```python
from build123d import *

# Parameters (mm, degrees)
CROQUIS2_R                = 19
SALIENTE_EXTRUIR1_DEPTH   = 39
CROQUIS3_W                = 25
CROQUIS3_H                = 35
SALIENTE_EXTRUIR2_DEPTH   = 53
CROQUIS4_R                = 3
CORTAR_EXTRUIR1_DEPTH     = 73.953752474
REDONDEO1_R               = 5
MATRIZC2_START            = 2
MATRIZC2_DEPTH            = 9.9999999
MATRIZC2_START_2          = 18.0000001
MATRIZC2_2_DEPTH          = 6.298293978
MATRIZC2_START_3          = 11.9999999
MATRIZC2_3_DEPTH          = 25.0000001
MATRIZC2_START_4          = -12.5
MATRIZC2_4_OUTLINE_R      = 3
MATRIZC2_4_DEPTH          = 25
MATRIZC2_5_OUTLINE_R      = 3
MATRIZC2_5_DEPTH          = 25
TALADRO_ROSCADO_3_4_102_D = 16.66748


with BuildPart() as part:
    # Croquis2 → Saliente-Extruir1 (new body)
    with BuildSketch(Plane(origin=(0, 0, 0), x_dir=(1, 0, 0), z_dir=(0, 1, 0))):
        with Locations(Location((0, 0, 0), (0, 0, 270))):
            Circle(CROQUIS2_R)
    extrude(amount=SALIENTE_EXTRUIR1_DEPTH)

    # Croquis3 → Saliente-Extruir2 (add)
    with BuildSketch(Plane.XY):
        with Locations((0, 19.5)):
            Rectangle(CROQUIS3_W, CROQUIS3_H)
    extrude(amount=SALIENTE_EXTRUIR2_DEPTH)

    # Croquis4 → Cortar-Extruir1 (cut, through all)
    with BuildSketch(Plane(origin=(12.5, 0, 0), x_dir=(0, 0, -1), z_dir=(1, 0, 0))):
        with Locations((-36, 15)):
            Circle(CROQUIS4_R)
        Polygon((-53, 27.185045424), (-53, 37), (-36, 37), align=None)
    extrude(amount=-CORTAR_EXTRUIR1_DEPTH, mode=Mode.SUBTRACT)

    # Redondeo1
    redondeo1_edges = [part.edges().sort_by_distance(p)[0] for p in [
        (12.5, 14.592522712, 53),
        (-12.5, 14.592522712, 53),
        (0, 27.185045424, 53),
        (0, 37, 36),
        (12.5, 19.5, 14.309088021),
        (-12.5, 19.5, 14.309088021),
    ]]
    fillet(redondeo1_edges, radius=REDONDEO1_R)

    # MatrizC2: read off the stored shape, not the designer's step
    # MatrizC2 outline → MatrizC2 (add)
    with BuildSketch(Plane(origin=(0, 0, 0), x_dir=(1, 0, 0), z_dir=(0, 1, 0)).offset(MATRIZC2_START)):
        with BuildLine():
            Line((-42.149346401, 32.995190528), (-49.649346401, 20.004809472))
            ThreePointArc((-49.649346401, 20.004809472), (-50.148848513, 16.210714247), (-47.819219382, 13.174682453))
            Line((-47.819219382, 13.174682453), (-18.642033731, -3.670773537))
            ThreePointArc((-18.642033731, -3.670773537), (-16.454482672, 9.5), (-6.142033731, 17.979861558))
            Line((-6.142033731, 17.979861558), (-35.319219382, 34.825317547))
            ThreePointArc((-35.319219382, 34.825317547), (-39.113314608, 35.32481966), (-42.149346401, 32.995190528))
        make_face()
        with BuildLine():
            ThreePointArc((6.142033731, 17.979861558), (16.454482672, 9.5), (18.642033731, -3.670773537))
            Line((18.642033731, -3.670773537), (47.819219382, 13.174682453))
            ThreePointArc((47.819219382, 13.174682453), (50.148848513, 16.210714247), (49.649346401, 20.004809472))
            Line((49.649346401, 20.004809472), (42.149346401, 32.995190528))
            ThreePointArc((42.149346401, 32.995190528), (39.113314608, 35.32481966), (35.319219382, 34.825317547))
            Line((35.319219382, 34.825317547), (6.142033731, 17.979861558))
        make_face()
    extrude(amount=MATRIZC2_DEPTH)

    # MatrizC2 2 outline → MatrizC2 2 (add)
    with BuildSketch(Plane(origin=(0, 0, 0), x_dir=(1, 0, 0), z_dir=(0, 1, 0)).offset(MATRIZC2_START_2)):
        with BuildLine():
            Line((-42.149346401, 32.995190528), (-49.649346401, 20.004809472))
            ThreePointArc((-49.649346401, 20.004809472), (-50.148848513, 16.210714247), (-47.819219382, 13.174682453))
            Line((-47.819219382, 13.174682453), (-18.642033731, -3.670773537))
            ThreePointArc((-18.642033731, -3.670773537), (-16.454482672, 9.5), (-6.142033731, 17.979861558))
            Line((-6.142033731, 17.979861558), (-35.319219382, 34.825317547))
            ThreePointArc((-35.319219382, 34.825317547), (-39.113314608, 35.32481966), (-42.149346401, 32.995190528))
        make_face()
        with BuildLine():
            ThreePointArc((6.142033731, 17.979861558), (16.454482672, 9.5), (18.642033731, -3.670773537))
            Line((18.642033731, -3.670773537), (47.819219382, 13.174682453))
            ThreePointArc((47.819219382, 13.174682453), (50.148848513, 16.210714247), (49.649346401, 20.004809472))
            Line((49.649346401, 20.004809472), (42.149346401, 32.995190528))
            ThreePointArc((42.149346401, 32.995190528), (39.113314608, 35.32481966), (35.319219382, 34.825317547))
            Line((35.319219382, 34.825317547), (6.142033731, 17.979861558))
        make_face()
    extrude(amount=MATRIZC2_2_DEPTH)

    # MatrizC2 3 outline → MatrizC2 3 (add)
    with BuildSketch(Plane(origin=(0, 0, 0), x_dir=(1, 0, 0), z_dir=(0, 1, 0)).offset(MATRIZC2_START_3)):
        with BuildLine():
            Line((-42.149346401, 32.995190528), (-49.649346401, 20.004809472))
            ThreePointArc((-49.649346401, 20.004809472), (-50.148848513, 16.210714247), (-47.819219382, 13.174682453))
            Line((-47.819219382, 13.174682453), (-18.642033731, -3.670773537))
            ThreePointArc((-18.642033731, -3.670773537), (-16.454482672, 9.5), (-6.142033731, 17.979861558))
            Line((-6.142033731, 17.979861558), (-35.319219382, 34.825317547))
            ThreePointArc((-35.319219382, 34.825317547), (-39.113314608, 35.32481966), (-42.149346401, 32.995190528))
        make_face()
        with BuildLine():
            ThreePointArc((6.142033731, 17.979861558), (16.454482672, 9.5), (18.642033731, -3.670773537))
            Line((18.642033731, -3.670773537), (47.819219382, 13.174682453))
            ThreePointArc((47.819219382, 13.174682453), (50.148848513, 16.210714247), (49.649346401, 20.004809472))
            Line((49.649346401, 20.004809472), (42.149346401, 32.995190528))
            ThreePointArc((42.149346401, 32.995190528), (39.113314608, 35.32481966), (35.319219382, 34.825317547))
            Line((35.319219382, 34.825317547), (6.142033731, 17.979861558))
        make_face()
    extrude(amount=MATRIZC2_3_DEPTH)

    # MatrizC2 4 outline → MatrizC2 4 (cut)
    with BuildSketch(Plane(origin=(0, 0, 0), x_dir=(0.8660254037844362, 0, -0.5000000000000042), z_dir=(0.5000000000000042, 0, 0.8660254037844363)).offset(MATRIZC2_START_4)):
        with BuildLine():
            ThreePointArc((34.660254038, 37), (35.954349263, 36.829629131), (37.160254038, 36.330127019))
            Line((37.160254038, 36.330127019), (50.5, 28.628421097))
            ThreePointArc((50.5, 28.628421097), (52.330127019, 26.798294078), (53, 24.298294078))
            Line((53, 24.298294078), (53.000000001, 37))
            Line((53.000000001, 37), (34.660254038, 37))
        make_face()
        with Locations((36, 15)):
            Circle(MATRIZC2_4_OUTLINE_R)
    extrude(amount=MATRIZC2_4_DEPTH, mode=Mode.SUBTRACT)

    # MatrizC2 5 outline → MatrizC2 5 (cut)
    with BuildSketch(Plane(origin=(0, 0, 0), x_dir=(0.8660254037844431, 0, 0.4999999999999921), z_dir=(0.4999999999999921, 0, -0.8660254037844433)).offset(MATRIZC2_START_4)):
        with BuildLine():
            ThreePointArc((-34.660254038, -37), (-35.954349263, -36.829629131), (-37.160254038, -36.330127019))
            Line((-37.160254038, -36.330127019), (-50.5, -28.628421097))
            ThreePointArc((-50.5, -28.628421097), (-52.330127019, -26.798294078), (-53, -24.298294078))
            Line((-53, -24.298294078), (-53, -37))
            Line((-53, -37), (-34.660254038, -37))
        make_face()
        with Locations((-36, -15)):
            Circle(MATRIZC2_5_OUTLINE_R)
    extrude(amount=MATRIZC2_5_DEPTH, mode=Mode.SUBTRACT)

    # Taladro roscado 3/4-102 (through all)
    with Locations(Plane.ZX.offset(39)):
        with Locations((0, 0)):
            Hole(TALADRO_ROSCADO_3_4_102_D / 2)


solid = part.part
```
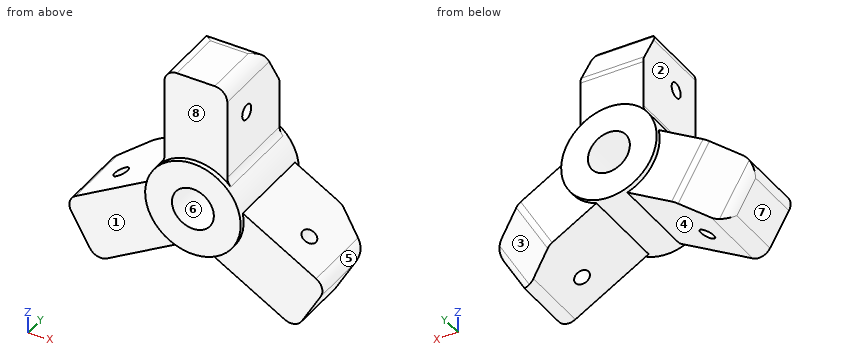
Here's how the part is built. I have some questions about the finished solid (model axes, mm). Face numbers are marked on the shaded views. A direction names the side the tool comes from. Give positions to 0.01 mm unless a question says otherwise; leave off trailing zeros. Loops run counter-clockwise (first coordinate to the right, second up) from the corner with the lowest first, then second, coordinate; pieces in that order, holes last. Notation, with made-up numbers: M 27.5,25 L 75.5,25 A25 cw 75.5,55 Z; hole C 10,24.5 d1. An arc over 180 degrees is marked long. Use one line per item in the form item = value. Start each with the question number.
Q1. If we section it at B-B (z = 0): Write out the boundary of the cut face in (x, y).
Q2. I need wall thicknesses on line 1 along X through (y, z) = (9, 28); line 2 along Y through (x, z) = (-1.5, 36); line 3 along X through (y, z) = (19, 7). Which ranges of each line are inside material? Lowest first, please.
Q3. If we section it at A-A (x = 0): Write out the boundary of the cut face in (y, z).
Q4. If we section it at C-C (y = 15): State how many separate pieces and enclosed holes the cut face has, then the cut area to 3 significant figures.
Q5. Which directions (+Z, -Z, +X, -X, +Y, -Y) give clear straight access to the entire face, cutting with the end or side of a thin tool? Please do the marked faces 1, 2, 3 and 4.
Q6. Thinking about a two-plate mould opening in X: for the marked faces 5, 6, 7 and 8, which applies, +X half, -X half, draft (parallel to the pull), parting line (faces both ways), or undercut?
Q7. Will these pins go through, and if not, where does the flat tip stop? pin 1 Ø4 at (x, y) = (1, 10.5) entering from -Z; pin 2 Ø6 at (y, z) = (20, 16) entering from +X; pin 3 Ø6.5 at (x, z) = (1.5, 25.5) entering from +Y; pin 4 Ø24 at (x, z) = (19.5, -6) entering from +Y.
Q8. If we section it at D-D (y = 25.5): Write out the boundary of the cut face in (x, z).
Taken from the geometry:
q1.outline = M -25,2 L -19,2 L -19,0 L -8.33,0 L -8.33,39 L -19,39 L -19,37 L -25,37 Z; M 8.33,0 L 19,0 L 19,2 L 25,2 L 25,37 L 19,37 L 19,39 L 8.33,39 Z
q2.line_1 = -12.5 to 12.5
q2.line_2 = 2 to 12, 18 to 36.82
q2.line_3 = -17.66 to -4.52, 4.52 to 17.66
q3.outline = M 0,-19 L 39,-19 L 39,-8.33 L 0,-8.33 Z; M 0,8.33 L 39,8.33 L 39,19 L 37,19 L 37,34.66 A5 ccw 36.33,37.16 L 28.63,50.5 A5 ccw 24.3,53 L 2,53 L 2,19 L 0,19 Z; hole C 15,36 d6
q4.separate_pieces = 4
q4.enclosed_holes = 1
q4.area = 3,100 mm^2
q5.face_1 = -Z, -X, -Y
q5.face_2 = +Z, -X, +Y, -Y
q5.face_3 = -Z, +X, +Y
q5.face_4 = -Z, +Y, -Y
q6.face_5 = +X half
q6.face_6 = undercut
q6.face_7 = -X half
q6.face_8 = draft
q7.pin_1 = -19
q7.pin_2 = 13.86
q7.pin_3 = 37
q7.pin_4 = 39
q8.outline = M -50.12,-18.89 L -41.42,-33.96 A5 ccw -35.32,-34.83 L -6.14,-17.98 A19 ccw 6.14,-17.98 L 35.32,-34.83 A5 ccw 41.42,-33.96 L 50.12,-18.89 A5 ccw 47.82,-13.17 L 18.64,3.67 A19 ccw 13.85,13 A5 cw 12.5,16.42 L 12.5,48 A5 ccw 8.7,52.85 L -8.7,52.85 A5 ccw -12.5,48 L -12.5,16.42 A5 cw -13.85,13 A19 ccw -18.64,3.67 L -47.82,-13.17 A5 ccw Z; hole C 0,0 d16.67
